Design review of the part shown in the three views and the two pictorial views. Dimensions are in mm from the part's minimum x, y and z. A direction names the side the tool comes from. Round coordinates to 2 decimals unless told otherwise and drop trailing zeros. Write each loop counter-clockwise with the first axis right and the second up, starting at its lowest first coordinate (ties: lowest second). Pieces come first, ordered by that corner, then holes. Notation, with made-up numbers: (25, 23.25) -> (49, 23.25) arc R16 ccw to (49, 52.25) -> close; hole circle Ø4 at (26, 45). An arc over 180 degrees is marked (long way). One line per question, with ' | ' between items. Start each with the question number.
1) For the marked faces 1 and 2, list the 3-axis set-ups (+Z, -Z, +X, -X, +Y, -Y) from which the entire face can be reached by the end or side of a thin tool; tool diameter is ignored.
2) Insertion check: pin 1 Ø5 at (x, z) = (141.5, 10) entering from +Y. The pin has a flat end and moves straight along its axis. Give the tip position at first contact, or say it passes through.
3) Mouldability with a two-part tool opening along Z and no side actions: class the marked faces 3, 4, 5 and 6 as +Z half, -Z half, draft (parallel to the pull), parting line (faces both ways), or undercut.
4) For probe 1 along Z at (x, y) = (9, 12); probe 2 along X at (y, z) = (10.5, 62); probe 3 along Z at (x, y) = (68, 32), list the stretches that pass through material, from the lowest coordinate up.
5) Consider section C-C (y = 20). Give the boundary of the cut face in (x, z).
6) Consider section B-B (z = 35.5). Give the boundary of the cut face in (x, y).
7) Consider section A-A (x = 129). Give the boundary of the cut face in (y, z).
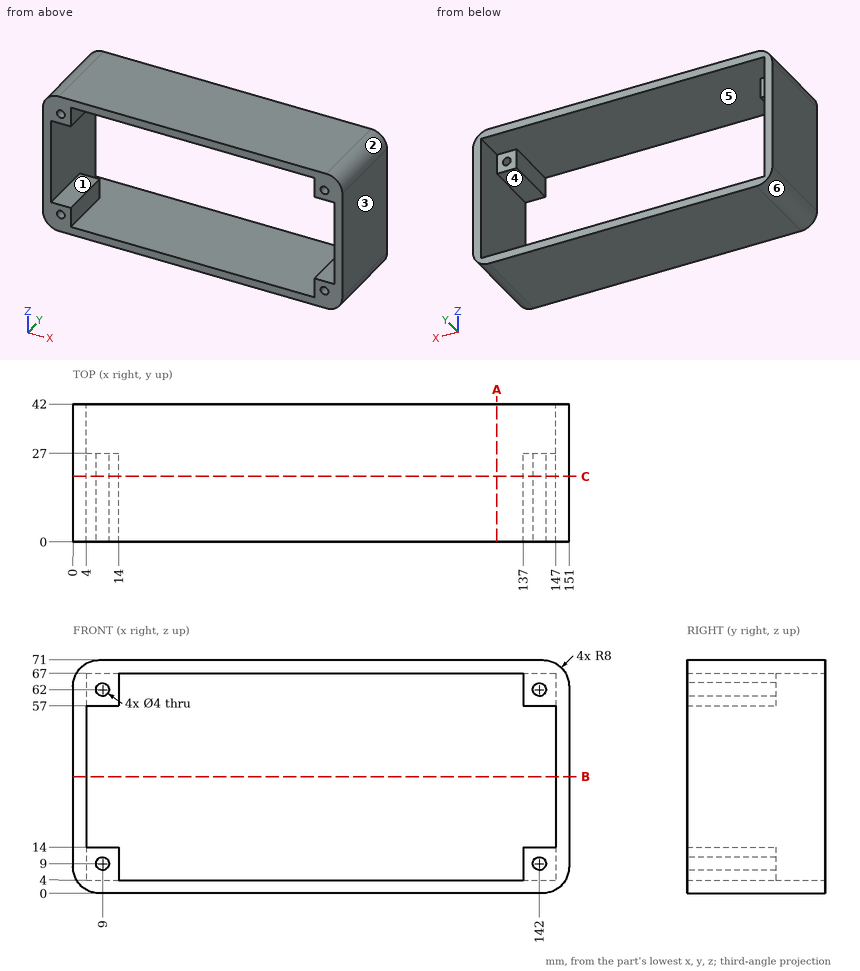
From the geometry:
1) face 1: +Y, -Y | face 2: +Z, +X, +Y, -Y
2) pin 1: stops at y = 27
3) face 3: draft | face 4: undercut | face 5: undercut | face 6: -Z half
4) probe 1: z = 0 to 7, 11 to 14, 57 to 60, 64 to 71 | probe 2: x = 0 to 7, 11 to 14, 137 to 140, 144 to 151 | probe 3: z = 0 to 4, 67 to 71
5) outline: (0, 8) arc R8 ccw to (8, 0) -> (143, 0) arc R8 ccw to (151, 8) -> (151, 63) arc R8 ccw to (143, 71) -> (8, 71) arc R8 ccw to (0, 63) -> close; hole (4, 14) -> (14, 14) -> (14, 4) -> (137, 4) -> (137, 14) -> (147, 14) -> (147, 57) -> (137, 57) -> (137, 67) -> (14, 67) -> (14, 57) -> (4, 57) -> close; hole circle Ø4 at (9, 9); hole circle Ø4 at (9, 62); hole circle Ø4 at (142, 9); hole circle Ø4 at (142, 62)
6) outline: (0, 0) -> (4, 0) -> (4, 42) -> (0, 42) -> close; (147, 0) -> (151, 0) -> (151, 42) -> (147, 42) -> close
7) outline: (0, 0) -> (42, 0) -> (42, 4) -> (0, 4) -> close; (0, 67) -> (42, 67) -> (42, 71) -> (0, 71) -> close
